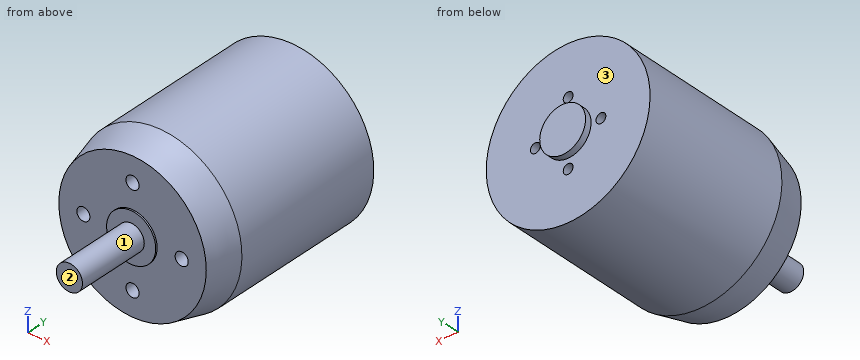
from build123d import *

# Parameters (mm, degrees)
F2_R     = 2
F3_DEPTH = 5
F4_R     = 7.5
F5_DEPTH = 0.5
F6_R     = 1.5
F7_DEPTH = 6


with BuildPart() as f1:
    # F0 (on Right) → F1 (revolve)
    with BuildSketch(Plane.YZ):
        Polygon((10, 25), (0, 22.5), (0, 4), (-23, 4), (-23, 0), (60, 0), (60, 7), (58, 7), (58, 25), align=None)
    revolve(axis=Axis((0, 18.5, 0), (0, 1, 0)))

    # F2 (on face) → F3 (cut)
    with BuildSketch(Plane.XZ):
        with Locations((15, 0)):
            Circle(F2_R)
        with Locations((0, 15)):
            Circle(F2_R)
        with Locations((-15, 0)):
            Circle(F2_R)
        with Locations((0, -15)):
            Circle(F2_R)
    extrude(amount=-F3_DEPTH, mode=Mode.SUBTRACT)

    # F4 (on face) → F5 (join)
    with BuildSketch(Plane.XZ):
        Circle(F4_R)
    extrude(amount=F5_DEPTH)

    # F6 (on face) → F7 (cut)
    with BuildSketch(Plane(origin=(0, 58, 0), x_dir=(-1, 0, 0), z_dir=(0, 1, 0))):
        with Locations((10, 0)):
            Circle(F6_R)
        with Locations((0, 10)):
            Circle(F6_R)
        with Locations((-10, 0)):
            Circle(F6_R)
        with Locations((0, -10)):
            Circle(F6_R)
    extrude(amount=-F7_DEPTH, mode=Mode.SUBTRACT)


solid = f1.part
Input: part model. Units: mm. Frame: model coordinates. Face numbers are marked on the shaded views. A direction names the side the tool comes from. Round coordinates to 2 decimals unless told otherwise and drop trailing zeros. Order: outer loops, then holes, each group sorted by start corner. A loop starts at its lowest first (then second) coordinate and runs counter-clockwise, first axis right, second up. Notation, with made-up numbers: (40, 88.25) - (56, 88.25) arc R12 ccw to (56, 111.25) - close; hole circle Ø5 at (46.25, -31). An arc over 180 degrees is marked (long way). Use a Markdown table: item, result.
1. Section A-A on y = 8. Return the cut outline in (x, z).
Evaluation:
| item | result |
|---|---|
| outline | circle Ø49 at (0, 0) |
2. First-contact query: pin 1 (2 mm diameter, centred on x = 16, z = 0.5, fed in from -Y); pin 2 (3.5 mm diameter, centred on x = -10, z = 0, fed in from +Y); pin 3 (3.5 mm diameter, centred on x = 0, z = 15, fed in from -Y). Flat tips, straight axial feed; report the tip coordinate or a pass-through.
Evaluation:
| item | result |
|---|---|
| pin 1 | y = 0 |
| pin 2 | y = 58 |
| pin 3 | y = 5 |
3. Section B-B on y = 34. Return the cut outline in (x, z).
Evaluation:
| item | result |
|---|---|
| outline | circle Ø50 at (0, 0) |
4. Access query for the marked faces 1, 2 and 3. Directions: +Z, -Z, +X, -X, +Y, -Y. A direction counts if a zero-diameter tool reaches every point of the face in a straight line with its end or side. Return the directions, or none.
Evaluation:
| item | result |
|---|---|
| face 1 | -Y |
| face 2 | +Z, -Z, +X, -X, -Y |
| face 3 | +Y |
5. Material intervals for probe 1 along Y at (x, z) = (16, 14.5); probe 2 along Z at (x, y) = (0, 1.85); probe 3 along Z at (x, y) = (15, 1.4), sorted ascending.
Evaluation:
| item | result |
|---|---|
| probe 1 | 0 to 58 |
| probe 2 | -22.96 to -17, -13 to 13, 17 to 22.96 |
| probe 3 | -17.24 to -2, 2 to 17.24 |
